from build123d import *

# Parameters (mm, degrees)
F1_DEPTH = 10
F2_DEPTH = 5


with BuildPart() as f1:
    # F0 (on Front) → F1 (new body)
    with BuildSketch(Plane.XZ):
        with BuildLine():
            ThreePointArc((0, -2.5), (1.767766953, -1.767766953), (2.5, 0))
            ThreePointArc((2.5, 0), (1.767766953, 1.767766953), (0, 2.5))
            Line((0, 2.5), (0, -2.5))
        make_face()
        with BuildLine():
            Line((0, -2.5), (0, 2.5))
            ThreePointArc((0, 2.5), (-2.5, 0), (0, -2.5))
        make_face()
    extrude(amount=F1_DEPTH)



with BuildPart() as f1b:
    # F0 (on Front) → F1, piece 2 (new body)
    with BuildSketch(Plane.XZ):
        with BuildLine():
            ThreePointArc((36.5, 0), (35.767766953, 1.767766953), (34, 2.5))
            Line((34, 2.5), (34, -2.5))
            ThreePointArc((34, -2.5), (35.767766953, -1.767766953), (36.5, 0))
        make_face()
        with BuildLine():
            Line((34, -2.5), (34, 2.5))
            ThreePointArc((34, 2.5), (31.5, 0), (34, -2.5))
        make_face()
    extrude(amount=F1_DEPTH)


with BuildPart() as f1c:
    # F0 (on Front) → F1, piece 3 (new body)
    with BuildSketch(Plane.XZ):
        with BuildLine():
            ThreePointArc((114, -2.5), (115.767766953, -1.767766953), (116.5, 0))
            Line((116.5, 0), (114, 0))
            Line((114, 0), (114, -2.5))
        make_face()
        with BuildLine():
            ThreePointArc((116.5, 0), (115.767766953, 1.767766953), (114, 2.5))
            Line((114, 2.5), (114, 0))
            Line((114, 0), (116.5, 0))
        make_face()
        with BuildLine():
            Line((114, 0), (114, 2.5))
            ThreePointArc((114, 2.5), (112.232233047, 1.767766953), (111.5, 0))
            Line((111.5, 0), (114, 0))
        make_face()
        with BuildLine():
            Line((114, 0), (111.5, 0))
            ThreePointArc((111.5, 0), (112.232233047, -1.767766953), (114, -2.5))
            Line((114, -2.5), (114, 0))
        make_face()
    extrude(amount=F1_DEPTH)


with BuildPart() as f1d:
    # F0 (on Front) → F1, piece 4 (new body)
    with BuildSketch(Plane.XZ):
        with BuildLine():
            Line((72, -2.5), (72, 2.5))
            ThreePointArc((72, 2.5), (69.5, 0), (72, -2.5))
        make_face()
        with BuildLine():
            ThreePointArc((74.5, 0), (73.767766953, 1.767766953), (72, 2.5))
            Line((72, 2.5), (72, -2.5))
            ThreePointArc((72, -2.5), (73.767766953, -1.767766953), (74.5, 0))
        make_face()
    extrude(amount=F1_DEPTH)


with BuildPart() as f1e:
    # F0 (on Front) → F1, piece 5 (new body)
    with BuildSketch(Plane.XZ):
        with BuildLine():
            ThreePointArc((116.5, -46), (114, -43.5), (111.5, -46))
            ThreePointArc((111.5, -46), (114, -48.5), (116.5, -46))
        make_face()
    extrude(amount=F1_DEPTH)


with BuildPart() as f1f:
    # F0 (on Front) → F1, piece 6 (new body)
    with BuildSketch(Plane.XZ):
        with BuildLine():
            Line((114, -96), (116.5, -96))
            ThreePointArc((116.5, -96), (115.767766953, -94.232233047), (114, -93.5))
            Line((114, -93.5), (114, -96))
        make_face()
        with BuildLine():
            Line((114, -96), (111.5, -96))
            ThreePointArc((111.5, -96), (112.232233047, -97.767766953), (114, -98.5))
            Line((114, -98.5), (114, -96))
        make_face()
        with BuildLine():
            ThreePointArc((114, -98.5), (115.767766953, -97.767766953), (116.5, -96))
            Line((116.5, -96), (114, -96))
            Line((114, -96), (114, -98.5))
        make_face()
        with BuildLine():
            Line((114, -96), (114, -93.5))
            ThreePointArc((114, -93.5), (112.232233047, -94.232233047), (111.5, -96))
            Line((111.5, -96), (114, -96))
        make_face()
    extrude(amount=F1_DEPTH)


with BuildPart() as f1g:
    # F0 (on Front) → F1, piece 7 (new body)
    with BuildSketch(Plane.XZ):
        with BuildLine():
            ThreePointArc((62.5, -96), (61.767766953, -94.232233047), (60, -93.5))
            Line((60, -93.5), (60, -98.5))
            ThreePointArc((60, -98.5), (61.767766953, -97.767766953), (62.5, -96))
        make_face()
        with BuildLine():
            Line((60, -98.5), (60, -93.5))
            ThreePointArc((60, -93.5), (57.5, -96), (60, -98.5))
        make_face()
    extrude(amount=F1_DEPTH)


with BuildPart() as f1h:
    # F0 (on Front) → F1, piece 8 (new body)
    with BuildSketch(Plane.XZ):
        with BuildLine():
            ThreePointArc((2, -98.5), (3.767766953, -97.767766953), (4.5, -96))
            Line((4.5, -96), (2, -96))
            Line((2, -96), (2, -98.5))
        make_face()
        with BuildLine():
            Line((2, -96), (-0.5, -96))
            ThreePointArc((-0.5, -96), (0.232233047, -97.767766953), (2, -98.5))
            Line((2, -98.5), (2, -96))
        make_face()
        with BuildLine():
            Line((2, -96), (2, -93.5))
            ThreePointArc((2, -93.5), (0.232233047, -94.232233047), (-0.5, -96))
            Line((-0.5, -96), (2, -96))
        make_face()
        with BuildLine():
            ThreePointArc((4.5, -96), (3.767766953, -94.232233047), (2, -93.5))
            Line((2, -93.5), (2, -96))
            Line((2, -96), (4.5, -96))
        make_face()
    extrude(amount=F1_DEPTH)


with BuildPart() as f1i:
    # F0 (on Front) → F1, piece 9 (new body)
    with BuildSketch(Plane.XZ):
        with BuildLine():
            ThreePointArc((-0.5, -158), (2, -160.5), (4.5, -158))
            Line((4.5, -158), (-0.5, -158))
        make_face()
        with BuildLine():
            Line((-0.5, -158), (4.5, -158))
            ThreePointArc((4.5, -158), (2, -155.5), (-0.5, -158))
        make_face()
    extrude(amount=F1_DEPTH)


with BuildPart() as f1_1:
    add(f1.part)

    add(f1b.part)  # F2 merges F1b

    add(f1c.part)  # F2 merges F1c

    add(f1d.part)  # F2 merges F1d

    add(f1e.part)  # F2 merges F1e

    add(f1f.part)  # F2 merges F1f

    add(f1g.part)  # F2 merges F1g

    add(f1h.part)  # F2 merges F1h

    add(f1i.part)  # F2 merges F1i
    # F0 (on Front) → F2 (join)
    with BuildSketch(Plane.XZ):
        with BuildLine():
            ThreePointArc((0, 2.5), (1.767766953, 1.767766953), (2.5, 0))
            ThreePointArc((2.5, 0), (1.767766953, -1.767766953), (0, -2.5))
            Line((0, -2.5), (34, -2.5))
            ThreePointArc((34, -2.5), (31.5, 0), (34, 2.5))
            Line((34, 2.5), (0, 2.5))
        make_face()
        with BuildLine():
            Line((72, 2.5), (34, 2.5))
            ThreePointArc((34, 2.5), (35.767766953, 1.767766953), (36.5, 0))
            ThreePointArc((36.5, 0), (35.767766953, -1.767766953), (34, -2.5))
            Line((34, -2.5), (72, -2.5))
            ThreePointArc((72, -2.5), (69.5, 0), (72, 2.5))
        make_face()
        with BuildLine():
            Line((114, -2.5), (111.5, -2.5))
            Line((111.5, -2.5), (111.5, -46))
            ThreePointArc((111.5, -46), (114, -43.5), (116.5, -46))
            Line((116.5, -46), (116.5, 0))
            ThreePointArc((116.5, 0), (115.767766953, -1.767766953), (114, -2.5))
        make_face()
        with BuildLine():
            Line((114, 2.5), (72, 2.5))
            ThreePointArc((72, 2.5), (73.767766953, 1.767766953), (74.5, 0))
            ThreePointArc((74.5, 0), (73.767766953, -1.767766953), (72, -2.5))
            Line((72, -2.5), (111.5, -2.5))
            Line((111.5, -2.5), (111.5, 0))
            ThreePointArc((111.5, 0), (112.232233047, 1.767766953), (114, 2.5))
        make_face()
        with BuildLine():
            ThreePointArc((116.5, -46), (114, -48.5), (111.5, -46))
            Line((111.5, -46), (111.5, -93.5))
            Line((111.5, -93.5), (114, -93.5))
            ThreePointArc((114, -93.5), (115.767766953, -94.232233047), (116.5, -96))
            Line((116.5, -96), (116.5, -46))
        make_face()
        with BuildLine():
            Line((111.5, -96), (111.5, -93.5))
            Line((111.5, -93.5), (60, -93.5))
            ThreePointArc((60, -93.5), (61.767766953, -94.232233047), (62.5, -96))
            ThreePointArc((62.5, -96), (61.767766953, -97.767766953), (60, -98.5))
            Line((60, -98.5), (114, -98.5))
            ThreePointArc((114, -98.5), (112.232233047, -97.767766953), (111.5, -96))
        make_face()
        with BuildLine():
            ThreePointArc((60, -98.5), (57.5, -96), (60, -93.5))
            Line((60, -93.5), (2, -93.5))
            ThreePointArc((2, -93.5), (3.767766953, -94.232233047), (4.5, -96))
            Line((4.5, -96), (4.5, -98.5))
            Line((4.5, -98.5), (60, -98.5))
        make_face()
        with BuildLine():
            Line((4.5, -158), (4.5, -98.5))
            Line((4.5, -98.5), (2, -98.5))
            ThreePointArc((2, -98.5), (0.232233047, -97.767766953), (-0.5, -96))
            Line((-0.5, -96), (-0.5, -158))
            ThreePointArc((-0.5, -158), (2, -155.5), (4.5, -158))
        make_face()
        with BuildLine():
            Line((2, -98.5), (4.5, -98.5))
            Line((4.5, -98.5), (4.5, -96))
            ThreePointArc((4.5, -96), (3.767766953, -97.767766953), (2, -98.5))
        make_face()
        with BuildLine():
            Line((111.5, 0), (111.5, -2.5))
            Line((111.5, -2.5), (114, -2.5))
            ThreePointArc((114, -2.5), (112.232233047, -1.767766953), (111.5, 0))
        make_face()
        with BuildLine():
            Line((114, -93.5), (111.5, -93.5))
            Line((111.5, -93.5), (111.5, -96))
            ThreePointArc((111.5, -96), (112.232233047, -94.232233047), (114, -93.5))
        make_face()
    extrude(amount=F2_DEPTH)


solid = f1_1.part
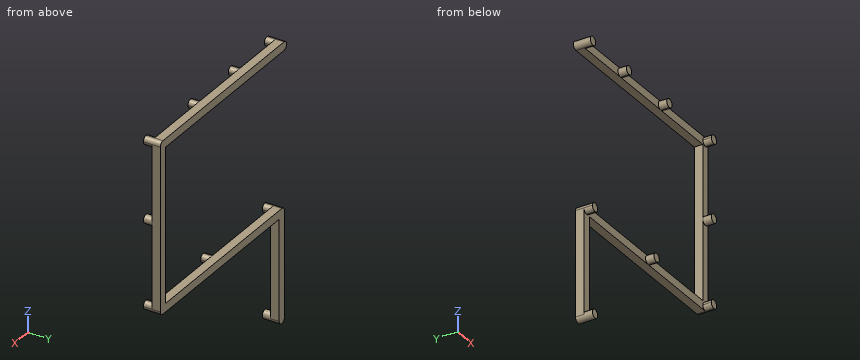
Verification items for the finished model (mm, model axes). Give positions to 0.01 mm unless a question says otherwise; leave off trailing zeros. Loops run counter-clockwise (first coordinate to the right, second up) from the corner with the lowest first, then second, coordinate; pieces in that order, holes last.
1) Sectioned sample at A-A, the plane x = 28.5. Enter the section's corners in (y, z), then the cut area to 3 significant figures.
2) Sectioned sample at C-C, the plane z = -109. Enter the section's corners in (x, y).
3) Depth check by flat-ended pin: pin 1 Ø6 at (x, y) = (52.5, -8.5) entering from +Z (3 decimals); pin 2 Ø5.5 at (y, z) = (-3, -123.5) entering from -X; pin 3 Ø1.5 at (x, z) = (13, -1) entering from -Y; pin 4 Ø5.5 at (y, z) = (-3.5, -117.5) entering from +X. Enter the tip coordinate at first touch or a pass-through.
4) Thickness scan on line 1 along Z through (x, y) = (112, -5.5); line 2 along Z through (x, y) = (54.5, -4.5); line 3 along X through (y, z) = (-0.25, -108). Record the ranges inside material, lowest first.
5) Sectioned sample at B-B, the plane y = -6.5. Count the separate pieces of the cut face and the enclosed holes in it, then the cut area to 3 significant figures.
Answers:
1. outline: (-5, -98.5) - (0, -98.5) - (0, -93.5) - (-5, -93.5) - close; (-5, -2.5) - (0, -2.5) - (0, 2.5) - (-5, 2.5) - close
1. area: 50.0 mm2
2. outline: (-0.5, -5) - (4.5, -5) - (4.5, 0) - (-0.5, 0) - close
3. pin 1: passes through
3. pin 2: stops at x = -0.5
3. pin 3: stops at y = -5
3. pin 4: stops at x = 4.5
4. line 1: z = -97.5 to -94.5, -47.5 to -44.5, -1.5 to 1.5
4. line 2: z = -98.5 to -93.5, -2.5 to 2.5
4. line 3: x = -0.5 to 4.5
5. separate pieces: 9
5. enclosed holes: 0
5. area: 177 mm2
